from build123d import *

# Parameters (mm, degrees)
EXTRUDE_1_DEPTH          = 50
CUT_EXTRUDE_1_DEPTH      = 10
CUT_EXTRUDE_1_DEPTH_BACK = 10
SKETCH_2_W               = 9.435028842
SKETCH_2_H               = 16.5


with BuildPart() as part:
    # Эскиз1 → Бобышка-Вытянуть1 (new body)
    with BuildSketch(Plane.XY):
        Polygon((2.867002202, -4.303564356), (2.867002202, -4.282485579), (5.867002202, -1.282485579), (11.302031044, -1.282485579), (11.302031044, 2.303564356), (2.867002202, 2.303564356), (-11.302031044, -4.303564356), align=None)
    extrude(amount=EXTRUDE_1_DEPTH)

    # Эскиз2 → Вырез-Вытянуть1 (cut, two sides: drawn at the far end of the back side and taken through both)
    with BuildSketch(Plane.XZ.offset(1.282485579).offset(-CUT_EXTRUDE_1_DEPTH_BACK)):
        with Locations((6.584516623, 25.063055317)):
            Rectangle(SKETCH_2_W, SKETCH_2_H)
    extrude(amount=CUT_EXTRUDE_1_DEPTH + CUT_EXTRUDE_1_DEPTH_BACK, mode=Mode.SUBTRACT)


solid = part.part
For this review, take the finished solid that the model builds, in its own axes (mm). A direction names the side the tool comes from. Coordinates: 2 decimals unless noted, no trailing zeros. Loops run counter-clockwise (first coordinate to the right, second up) from the corner with the lowest first, then second, coordinate; pieces in that order, holes last. Notation, with made-up numbers: (58.5, -12.5) - (103.5, -12.5) arc R11 ccw to (103.5, 3.5) - close; hole circle Ø4 at (67, 18.5). An arc over 180 degrees is marked (long way). Use a Markdown table: item, result. Add a question column.
Item 1: Tool access review of faces 1 (the face through (5, 0, 16.813)), 2 (the face through (2, -1, 50)), 3 (the face through (9, -1.282, 8)): name each direction out of +Z, -Z, +X, -X, +Y, -Y from which nothing blocks a thin tool from reaching the whole face with its end or side.
Item 2: Mouldability with a two-part tool opening along Z and no side actions: class faces 4 (the face through (7, 2.304, 42)), 5 (the face through (5, 0, 33.313)), 6 (the face through (2, -1, 0)) as pulls with the +Z half, pulls with the -Z half, needs draft (parallel to the pull), parting line crosses it, or undercut.
Item 3: For line 1 (Z direction, x = 3.25, y = 0.75); line 2 (Y direction, x = 9.25, z = 9); line 3 (X direction, y = -3.25, z = 9), list the stretches that pass through material, from the lowest coordinate up.
Item 4: We need section C-C (y = 1). Give the boundary of the cut face in (x, z).
Item 5: Insertion check: pin 1 Ø2.5 at (x, z) = (9, 5) entering from -Y; pin 2 Ø3 at (y, z) = (-2.5, 18.5) entering from -X. Each pin has a flat end and moves straight along its axis. Give the tip position at first contact, or say it passes through.
Item 6: We need section A-A (x = 6.5). Give the boundary of the cut face in (y, z).
Item 7: We need section D-D (y = -3). Give the boundary of the cut face in (x, z), and give its area (3 significant figures).
Results list:
| question | item | result |
|---|---|---|
| 1 | face 1 | +X, +Y, -Y |
| 1 | face 2 | +Z, +X, -X, +Y, -Y |
| 1 | face 3 | +Z, -Z, +X, -Y |
| 2 | face 4 | needs draft |
| 2 | face 5 | undercut |
| 2 | face 6 | pulls with the -Z half |
| 3 | line 1 | z = 0 to 16.81, 33.31 to 50 |
| 3 | line 2 | y = -1.28 to 2.3 |
| 3 | line 3 | x = -9.04 to 3.9 |
| 4 | outline | (0.07, 0) - (11.3, 0) - (11.3, 16.81) - (1.87, 16.81) - (1.87, 33.31) - (11.3, 33.31) - (11.3, 50) - (0.07, 50) - close |
| 5 | pin 1 | stops at y = -1.28 |
| 5 | pin 2 | stops at x = -10.65 |
| 6 | outline | (-1.28, 0) - (2.3, 0) - (2.3, 16.81) - (-1.28, 16.81) - close; (-1.28, 33.31) - (2.3, 33.31) - (2.3, 50) - (-1.28, 50) - close |
| 7 | outline | (-8.51, 0) - (4.15, 0) - (4.15, 16.81) - (1.87, 16.81) - (1.87, 33.31) - (4.15, 33.31) - (4.15, 50) - (-8.51, 50) - close |
| 7 | area | 595 mm^2 |
